Part model, mm, in its own coordinate system. Face numbers are marked on the shaded views. A direction names the side the tool comes from. Give positions to 0.01 mm unless a question says otherwise; leave off trailing zeros. Order: outer loops, then holes, each group sorted by start corner. A loop starts at its lowest first (then second) coordinate and runs counter-clockwise, first axis right, second up. Notation, with made-up numbers: (75.25, 33) - (125.25, 33) arc R20 cw to (125.25, 47) - close; hole circle Ø1 at (66, 56.5). An arc over 180 degrees is marked (long way). Use a Markdown table: item, result. Add a question column.
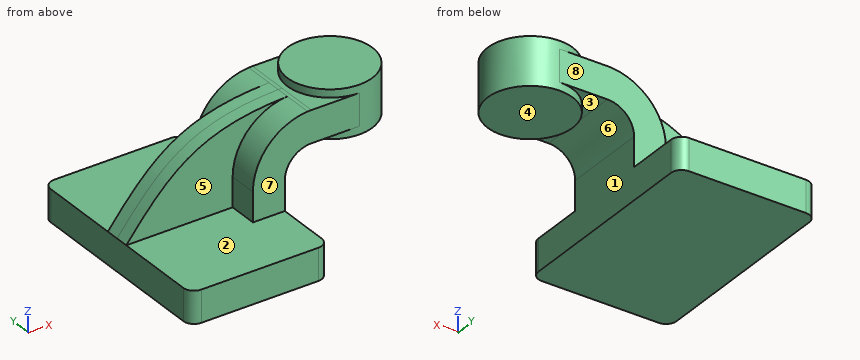
from build123d import *

# Parameters (mm, degrees)
F1_DEPTH = 63.5
F2_DEPTH = 25.4
F3_DEPTH = 7.9375
F0_W     = 25.4
F0_H     = 19.05
F4_DEPTH = 25.4
F6_R     = 6.35


with BuildPart() as f1:
    # F0 (on Front) → F1 (new body, symmetric)
    with BuildSketch(Plane.XZ):
        Polygon((22.225, 9.525), (-41.275, 9.525), (-41.275, -9.525), (41.275, -9.525), (41.275, 9.525), align=None)
    extrude(amount=F1_DEPTH, both=True)

    # F0 (on Front) → F2 (join, symmetric)
    with BuildSketch(Plane.XZ):
        with BuildLine():
            Line((22.225, 27.0002), (22.225, 9.525))
            Line((22.225, 9.525), (41.275, 9.525))
            Line((41.275, 9.525), (41.275, 27.0002))
            ThreePointArc((41.275, 27.0002), (45.9246798487, 38.2255201513), (57.15, 42.8752))
            Line((57.15, 42.8752), (60.325, 42.8752))
            Line((60.325, 42.8752), (60.325, 61.9252))
            Line((60.325, 61.9252), (57.15, 61.9252))
            add(Edge.make_bspline(
                [(54.9309637921, 61.854633051), (55.6637542078, 61.8810124388), (56.4033914289, 61.9045304692), (57.15, 61.9252)],
                knots=[109.9388089339, 109.9388089339, 109.9388089339, 109.9388089339, 111.5045361635, 111.5045361635, 111.5045361635, 111.5045361635], degree=3))
            ThreePointArc((54.9309637921, 61.854633051), (31.6818290354, 50.8984822127), (22.225, 27.0002))
        make_face()
    extrude(amount=F2_DEPTH, both=True)

    # F0 (on Front) → F3 (join, symmetric)
    with BuildSketch(Plane.XZ):
        with BuildLine():
            add(Edge.make_bspline(
                [(-41.275, 9.525), (-14.2194517609, 44.0428960459), (3.4774896668, 60.0023829163), (54.9309637921, 61.854633051)],
                knots=[0, 0, 0, 0, 109.9388089339, 109.9388089339, 109.9388089339, 109.9388089339], degree=3))
            Line((-41.275, 9.525), (22.225, 9.525))
            Line((22.225, 9.525), (22.225, 27.0002))
            ThreePointArc((22.225, 27.0002), (31.6818290354, 50.8984822127), (54.9309637921, 61.854633051))
        make_face()
    extrude(amount=F3_DEPTH, both=True)

    # F0 (on Front) → F4 (join, symmetric)
    with BuildSketch(Plane.XZ):
        with Locations((73.025, 52.4002)):
            Rectangle(F0_W, F0_H)
    extrude(amount=F4_DEPTH, both=True)

    # F0 (on Front) → F5 (revolve)
    with BuildSketch(Plane.XZ):
        Polygon((85.725, 66.675), (85.725, 61.9252), (85.725, 42.8752), (85.725, 38.1), (111.125, 38.1), (111.125, 66.675), align=None)
    revolve(axis=Axis((85.725, 0, 52.3875), (0, 0, 1)))

    # F6
    f6_edges = [f1.edges().sort_by_distance(p)[0] for p in [
        (41.275, -63.5, 0),
        (-41.275, -63.5, 0),
        (41.275, 63.5, 0),
        (-41.275, 63.5, 0),
    ]]
    fillet(f6_edges, radius=F6_R)


solid = f1.part
1. Mould opens along X. For the marked faces 1, 2 and 3 say: released by +X, released by -X, zero draft, split by the parting line, or undercut.
2. Cut at B-B (x = 79). Write the cut outline in (y, z) (3 decimals), plus the area to 3 significant figures.
3. Cut at A-A (y = -28). Write the cut outline in (x, z) (3 decimals).
4. Pin check, flat tips, straight feed: P1, Ø23, axis at x = 76, y = -4.5, coming from the -Z side; P2, Ø12, axis at x = 31.5, y = 44, coming from the +Z side (3 decimals); P3, Ø8.5, axis at y = -18.5, z = 19.5, coming from the -X side (3 decimals). Stop position of each tip, or through.
5. Drill centre lines: probe 1 along Y at (x, z) = (80.5, 61); probe 2 along Z at (x, y) = (91, 4.5) (3 decimals); probe 3 along Z at (x, y) = (-14.5, 23.5) (3 decimals). Where is each one in solid material? Low to high. Write a range as [from, to].
6. Tool access for the marked faces 4, 5, 6, 7 and 8: list every direction of +Z, -Z, +X, -X, +Y, -Y with a clear straight run to the whole face (end or side of a thin tool).
Responses:
| question | item | result |
|---|---|---|
| 1 | face 1 | released by +X |
| 1 | face 2 | zero draft |
| 1 | face 3 | undercut |
| 2 | outline | (-25.4, 42.875) - (-24.494, 42.875) - (-24.494, 38.1) - (24.494, 38.1) - (24.494, 42.875) - (25.4, 42.875) - (25.4, 61.925) - (24.494, 61.925) - (24.494, 66.675) - (-24.494, 66.675) - (-24.494, 61.925) - (-25.4, 61.925) - close |
| 2 | area | 1,430 mm² |
| 3 | outline | (-41.275, -9.525) - (41.275, -9.525) - (41.275, 9.525) - (-41.275, 9.525) - close |
| 4 | P1 | stops at z = 38.1 |
| 4 | P2 | stops at z = 9.525 |
| 4 | P3 | stops at x = 22.225 |
| 5 | probe 1 | y = [-25.4, 25.4] |
| 5 | probe 2 | z = [38.1, 66.675] |
| 5 | probe 3 | z = [-9.525, 9.525] |
| 6 | face 4 | -Z, +X, +Y, -Y |
| 6 | face 5 | +Z, -X, -Y |
| 6 | face 6 | -Z, +Y, -Y |
| 6 | face 7 | +Z, +X, -X, -Y |
| 6 | face 8 | +Z, +X, -X, +Y |
